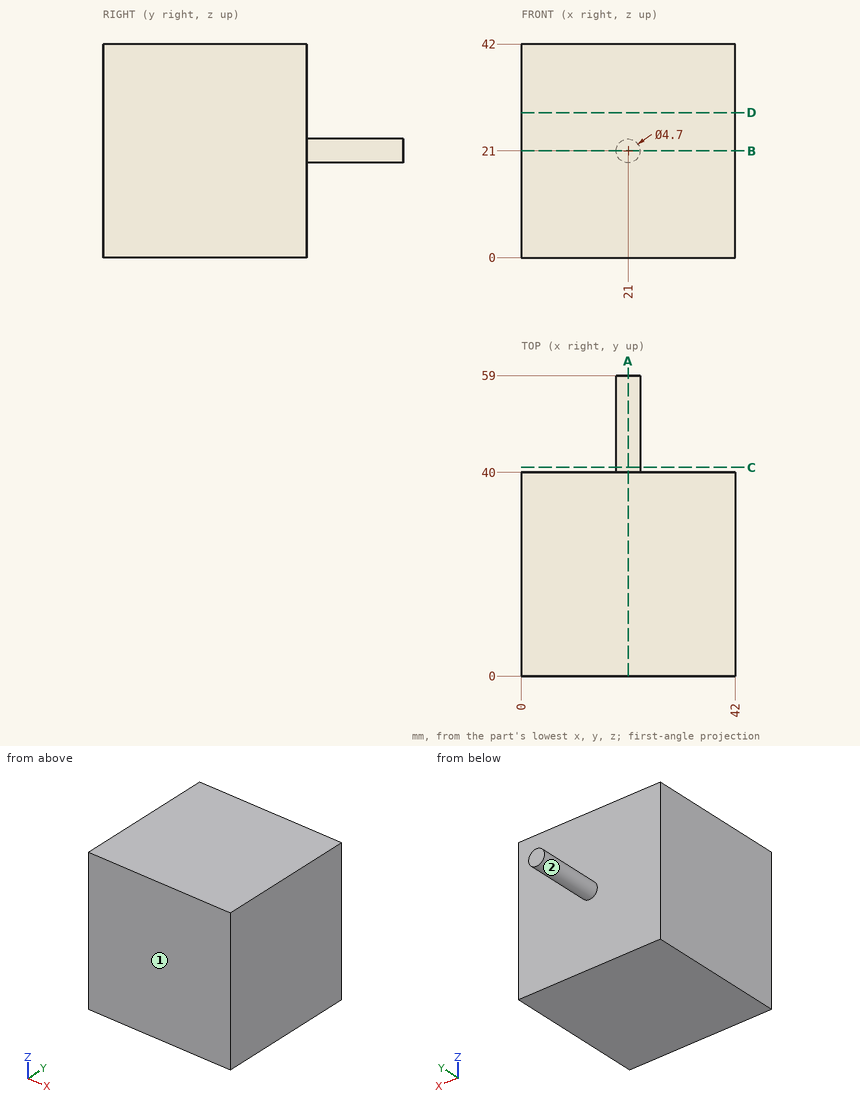
Geometry check sheet. Reference: drawing and pictorial views, mm from the part's lowest x, y, z. A direction names the side the tool comes from. Give positions to 0.01 mm unless a question says otherwise; leave off trailing zeros. Order: outer loops, then holes, each group sorted by start corner. A loop starts at its lowest first (then second) coordinate and runs counter-clockwise, first axis right, second up. Notation, with made-up numbers: (56.25, 9) -> (106.25, 9) arc R19 cw to (106.25, 26) -> close; hole circle Ø11 at (-8, -26.5). An arc over 180 degrees is marked (long way). Use CSV: the item, a comma, the result in double quotes. Start each with the question number.
1) Sectioned sample at C-C, the plane y = 41. Record the boundary of the cut face in (x, z).
2) Set-up check for the marked faces 1 and 2: record each of +Z, -Z, +X, -X, +Y, -Y from which the full face is reachable in a straight line by a thin tool's end or side.
3) Sectioned sample at B-B, the plane z = 21. Record the boundary of the cut face in (x, y).
4) Go/stop test with a flat-tipped pin: P1, Ø3, axis at x = 37.5, z = 34.5, coming from the +Y side. Record where the tip stops, or that it passes through.
5) Sectioned sample at A-A, the plane x = 21. Record the boundary of the cut face in (y, z).
6) Material ranges on line 1 (Y direction, x = 33.5, z = 20.5); line 2 (X direction, y = 52, z = 22.5), recorded low to high. Write a range as from..to.
7) Sectioned sample at D-D, the plane z = 28.5. Record the boundary of the cut face in (x, y), plus the area to 3 significant figures.
Recorded:
1,outline,"circle Ø4.7 at (21, 21)"
2,face 1,"+Z, -Z, +X, -X, -Y"
2,face 2,"+Y"
3,outline,"(0, 0) -> (42, 0) -> (42, 40) -> (23.35, 40) -> (23.35, 59) -> (18.65, 59) -> (18.65, 40) -> (0, 40) -> close"
4,P1,"y = 40"
5,outline,"(0, 0) -> (40, 0) -> (40, 18.65) -> (59, 18.65) -> (59, 23.35) -> (40, 23.35) -> (40, 42) -> (0, 42) -> close"
6,line 1,"0..40"
6,line 2,"19.19..22.81"
7,outline,"(0, 0) -> (42, 0) -> (42, 40) -> (0, 40) -> close"
7,area,"1,680 mm2"
